```python
from build123d import *

# Parameters (mm, degrees)
ESQUISSE_BASE_CODEUR_R    = 19.25
BASE_CODEUR_DEPTH         = 33.5
ESQUISSE_PLATEAU_CODEUR_R = 10
PLATEAU_CODEUR_DEPTH      = 5
ESQUISSE_ARBRE_R          = 3
ARBRE_DEPTH               = 15
USINAGE_ARBRE_DEPTH       = 12


with BuildPart() as part:
    # esquisse_base_codeur → base_codeur (new body)
    with BuildSketch(Plane(origin=(0, 0, 0), x_dir=(0, 0, -1), z_dir=(1, 0, 0))):
        Circle(ESQUISSE_BASE_CODEUR_R)
    extrude(amount=BASE_CODEUR_DEPTH)

    # esquisse_plateau_codeur → plateau_codeur (add)
    with BuildSketch(Plane(origin=(33.5, 0, 0), x_dir=(0, 0, -1), z_dir=(1, 0, 0))):
        Circle(ESQUISSE_PLATEAU_CODEUR_R)
    extrude(amount=PLATEAU_CODEUR_DEPTH)

    # esquisse_arbre → arbre (add)
    with BuildSketch(Plane(origin=(38.5, 0, 0), x_dir=(0, 0, -1), z_dir=(1, 0, 0))):
        Circle(ESQUISSE_ARBRE_R)
    extrude(amount=ARBRE_DEPTH)

    # esquisse_usinage_arbre → usinage_arbre (cut)
    with BuildSketch(Plane(origin=(53.5, 0, 0), x_dir=(0, 0, -1), z_dir=(1, 0, 0))):
        with BuildLine():
            Line((-1.658312395, 2.5), (1.658312395, 2.5))
            ThreePointArc((1.658312395, 2.5), (0, 3), (-1.658312395, 2.5))
        make_face()
    extrude(amount=-USINAGE_ARBRE_DEPTH, mode=Mode.SUBTRACT)


solid = part.part
```
Could you check a few things on this model? Use its own coordinates, in mm. A direction names the side the tool comes from. Coordinates: 2 decimals unless noted, no trailing zeros. Loops run counter-clockwise (first coordinate to the right, second up) from the corner with the lowest first, then second, coordinate; pieces in that order, holes last. Notation, with made-up numbers: M 88,-40 L 97,-40 A33 cw 97,-6 Z; hole C 83,4.5 d1. An arc over 180 degrees is marked long. Put each result on its own line as item: value. Start each with the question number.
(1) Suppose I cut it at D-D on z = 5. Please give me the cut outline in (x, y).
(2) For faces 1 (the face through (53.5, 0, 0)), 2 (the face through (45.9, -2.93, 0.65)), 3 (the face through (48, 2.5, 0)), which set-ups out of +Z, -Z, +X, -X, +Y, -Y let a thin tool reach every point of the face, with its end or its side?
(3) Suppose I cut it at A-A on z = 0. Please give me the cut outline in (x, y), then the cut area to 3 significant figures.
(4) Suppose I cut it at C-C on x = 23. Please give me the cut outline in (y, z), then the cut area to 3 significant figures.
(5) Suppose I cut it at B-B on y = 0. Please give me the cut outline in (x, z), then the cut area to 3 significant figures.
(6) Will these pins go through, and if not, where does the flat tip stop? P1, Ø5, axis at y = -3, z = -5.5, coming from the +X side; P2, Ø1, axis at x = 46, z = 0.5, coming from the +Y side; P3, Ø1.5, axis at x = 28, z = 5, coming from the +Y side (3 decimals).
(7) I need wall thicknesses on line 1 (Z direction, x = 22.5, y = 0.5); line 2 (X direction, y = 8.5, z = -3.5); line 3 (X direction, y = 8, z = 7). Which ranges of each line are inside material? Lowest first, please. Write a range as from..to.
Solutions:
1. outline: M 0,-18.59 L 33.5,-18.59 L 33.5,-8.66 L 38.5,-8.66 L 38.5,8.66 L 33.5,8.66 L 33.5,18.59 L 0,18.59 Z
2. face 1: +Z, -Z, +X, +Y, -Y
2. face 2: +X
2. face 3: +Z, -Z, +X, +Y
3. outline: M 0,-19.25 L 33.5,-19.25 L 33.5,-10 L 38.5,-10 L 38.5,-3 L 53.5,-3 L 53.5,2.5 L 41.5,2.5 L 41.5,3 L 38.5,3 L 38.5,10 L 33.5,10 L 33.5,19.25 L 0,19.25 Z
3. area: 1,470 mm2
4. outline: C 0,0 d38.5
4. area: 1,160 mm2
5. outline: M 0,-19.25 L 33.5,-19.25 L 33.5,-10 L 38.5,-10 L 38.5,-3 L 53.5,-3 L 53.5,3 L 38.5,3 L 38.5,10 L 33.5,10 L 33.5,19.25 L 0,19.25 Z
5. area: 1,480 mm2
6. P1: stops at x = 38.5
6. P2: stops at y = 2.5
6. P3: stops at y = 18.775
7. line 1: z = -19.24..19.24
7. line 2: x = 0..38.5
7. line 3: x = 0..33.5
